Geometry: final body of the model. Coordinates: model frame, mm. Face numbers are marked on the shaded views. Round coordinates to 2 decimals unless told otherwise and drop trailing zeros. Loops run counter-clockwise (first coordinate to the right, second up) from the corner with the lowest first, then second, coordinate; pieces in that order, holes last. Notation, with made-up numbers: (-7, -3) - (28, -3) arc R24 cw to (28, 9) - close; hole circle Ø8 at (72, 3.5). An arc over 180 degrees is marked (long way). Answer in a Markdown table with one row per item. Add a question column.
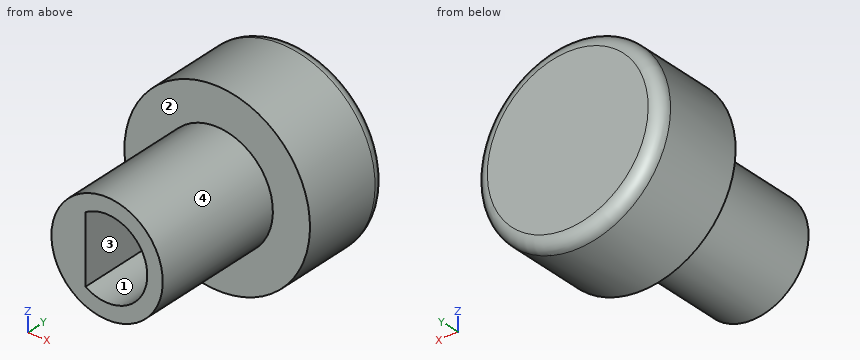
from build123d import *

# Parameters (mm, degrees)
SKETCH1_R           = 7.5
BOSS_EXTRUDE1_DEPTH = 7.5
FILLET1_R           = 1
SKETCH2_R           = 4.5
BOSS_EXTRUDE2_DEPTH = 11
SKETCH3_R           = 3.25
CUT_EXTRUDE1_DEPTH  = 11
BOSS_EXTRUDE3_START = 11
BOSS_EXTRUDE3_DEPTH = 11


with BuildPart() as part:
    # Sketch1 → Boss-Extrude1 (new body)
    with BuildSketch(Plane(origin=(0, 0, 0), x_dir=(1, 0, 0), z_dir=(0, 1, 0))):
        with Locations(Location((0, 0, 0), (0, 0, 270))):
            Circle(SKETCH1_R)
    extrude(amount=BOSS_EXTRUDE1_DEPTH)

    # Fillet1
    fillet1_edges = [part.edges().sort_by_distance(p)[0] for p in [
        (0, 7.5, -7.5),
    ]]
    fillet(fillet1_edges, radius=FILLET1_R)

    # Sketch2 → Boss-Extrude2 (add)
    with BuildSketch(Plane.XZ):
        with Locations(Location((0, 0, 0), (0, 0, 270))):
            Circle(SKETCH2_R)
    extrude(amount=BOSS_EXTRUDE2_DEPTH)

    # Sketch3 → Cut-Extrude1 (cut)
    with BuildSketch(Plane(origin=(0, -11, 0), x_dir=(-1, 0, 0), z_dir=(0, -1, 0))):
        with Locations(Location((0, 0, 0), (0, 0, 90))):
            Circle(SKETCH3_R)
    extrude(amount=-CUT_EXTRUDE1_DEPTH, mode=Mode.SUBTRACT)

    # Sketch4 → Boss-Extrude3 (add)
    with BuildSketch(Plane(origin=(0, 0, 0), x_dir=(-1, 0, 0), z_dir=(0, -1, 0)).offset(BOSS_EXTRUDE3_START)):
        with BuildLine():
            Line((1.75, 2.738612788), (1.75, -2.738612788))
            ThreePointArc((1.75, -2.738612788), (2.850438563, -1.5612495), (3.25, 0))
            ThreePointArc((3.25, 0), (2.850438563, 1.5612495), (1.75, 2.738612788))
        make_face()
    extrude(amount=-BOSS_EXTRUDE3_DEPTH)


solid = part.part
1) Contact query for flat-ended pins moving along their axis: pin 1 Ø4 at (x, y) = (6, -2.5) entering from +Z; pin 2 Ø4 at (x, y) = (3.5, -8) entering from +Z; pin 3 Ø1 at (y, z) = (0, 4.5) entering from +X; pin 4 Ø1.5 at (x, y) = (5.5, -3.5) entering from +Z. Output: stop coordinate, or through.
2) Section C-C, the plane y = -9. Return the cut outline in (x, z), and give its area (3 significant figures).
3) Section B-B, the plane z = 0. Return the cut outline in (x, y), and give its area (3 significant figures).
4) Pull-direction query (X, two-part tool) for the marked faces 1, 2, 3 and 4; classes: pulls with the +X half, pulls with the -X half, needs draft (parallel to the pull), parting line crosses it, or undercut.
5) Section A-A, the plane x = 0. Return the cut outline in (y, z).
6) Material intervals for line 1 along X through (y, z) = (-2.75, 0); line 2 along Y through (x, z) = (3, -0.5); line 3 along X through (y, z) = (-3, 1.25), sorted ascending. Write a range as from..to.
Evaluation:
| question | item | result |
|---|---|---|
| 1 | pin 1 | stops at z = 2.06 |
| 1 | pin 2 | stops at z = 4.24 |
| 1 | pin 3 | stops at x = 6.34 |
| 1 | pin 4 | passes through |
| 2 | outline | circle Ø9 at (0, 0); hole (-1.75, -2.74) arc R3.25 ccw (long way) to (-1.75, 2.74) - close |
| 2 | area | 36.2 mm² |
| 3 | outline | (-7.5, 0) - (-4.5, 0) - (-4.5, -11) - (-1.75, -11) - (-1.75, 0) - (3.25, 0) - (3.25, -11) - (4.5, -11) - (4.5, 0) - (7.5, 0) - (7.5, 6.5) arc R1 ccw to (6.5, 7.5) - (-6.5, 7.5) arc R1 ccw to (-7.5, 6.5) - close |
| 3 | area | 156 mm² |
| 4 | face 1 | undercut |
| 4 | face 2 | needs draft |
| 4 | face 3 | undercut |
| 4 | face 4 | parting line crosses it |
| 5 | outline | (-11, -4.5) - (0, -4.5) - (0, -7.5) - (6.5, -7.5) arc R1 ccw to (7.5, -6.5) - (7.5, 6.5) arc R1 ccw to (6.5, 7.5) - (0, 7.5) - (0, 4.5) - (-11, 4.5) - (-11, 3.25) - (0, 3.25) - (0, -3.25) - (-11, -3.25) - close |
| 6 | line 1 | x = -4.5..-1.75, 3.25..4.5 |
| 6 | line 2 | y = 0..7.5 |
| 6 | line 3 | x = -4.32..-1.75, 3..4.32 |
